from build123d import *

# Parameters (mm, degrees)
SKETCH1_W                        = 132.5
SKETCH1_H                        = 117
BOSS_EXTRUDE1_DEPTH              = 55.25
CUT_EXTRUDE1_REACH               = 147.364
SKETCH3_W                        = 39
SKETCH3_H                        = 37.83
CUT_EXTRUDE2_DEPTH               = 85
SKETCH4_W                        = 20.6
SKETCH4_H                        = 13
BOSS_EXTRUDE2_DEPTH              = 32
SKETCH5_W                        = 27.5
SKETCH5_H                        = 68.25
CUT_EXTRUDE3_DEPTH               = 3
SKETCH6_W                        = 46.9
SKETCH6_H                        = 3.4
CUT_EXTRUDE4_DEPTH               = 46.9
SKETCH8_R                        = 4.2
SKETCH8_R_2                      = 4.5
CUT_EXTRUDE5_DEPTH               = 14
SKETCH9_R                        = 14.58
CUT_EXTRUDE6_DEPTH               = 15.3
SKETCH10_R                       = 11.2
CUT_EXTRUDE7_DEPTH               = 7.22
BOSS_EXTRUDE3_DEPTH              = 4.25
CUT_EXTRUDE8_REACH               = 116.313
CUT_EXTRUDE8_END_RADIUS          = 4.2
SKETCH15_R                       = 2
F_4_0_MM_DOWEL_HOLES1_D          = 4
F_4_0_MM_DOWEL_HOLES2_AT_2_COUNT = 2
F_4_0_MM_DOWEL_HOLES2_AT_2_PITCH = 30
F_4_0_MM_DOWEL_HOLES3_D          = 4
F_4_0_MM_DOWEL_HOLES3_DEPTH      = 10
F_4_0_MM_DOWEL_HOLES3_TIP        = 1.201721238


with BuildPart() as part:
    # Sketch1 → Boss-Extrude1 (new body)
    with BuildSketch(Plane.XY):
        Rectangle(SKETCH1_W, SKETCH1_H)
    extrude(amount=BOSS_EXTRUDE1_DEPTH)

    # Sketch2 → Cut-Extrude1 (cut, up to next)
    with BuildSketch(Plane(origin=(0, 58.5, 0), x_dir=(1, 0, 0), z_dir=(0, 1, 0)), mode=Mode.PRIVATE) as cut_extrude1_sk1:
        with BuildLine():
            Line((-57.7, -32), (-57.7, -55.25))
            Line((-57.7, -55.25), (-22.3, -55.25))
            Line((-22.3, -55.25), (-22.3, -32))
            ThreePointArc((-22.3, -32), (-40, -14.3), (-57.7, -32))
        make_face()
    cut_extrude1_tool1 = extrude(cut_extrude1_sk1.sketch, amount=-CUT_EXTRUDE1_REACH, mode=Mode.PRIVATE) & part.part
    # Sketch2 → Cut-Extrude1 (cut, up to next)
    with BuildSketch(Plane(origin=(0, 58.5, 0), x_dir=(1, 0, 0), z_dir=(0, 1, 0)), mode=Mode.PRIVATE) as cut_extrude1_sk2:
        with BuildLine():
            Line((57.7, -32), (57.7, -55.25))
            Line((57.7, -55.25), (22.3, -55.25))
            Line((22.3, -55.25), (22.3, -32))
            ThreePointArc((22.3, -32), (40, -14.3), (57.7, -32))
        make_face()
    cut_extrude1_tool2 = extrude(cut_extrude1_sk2.sketch, amount=-CUT_EXTRUDE1_REACH, mode=Mode.PRIVATE) & part.part
    add(cut_extrude1_tool1.solids().sort_by_distance((-40, 58.5, 36.464181))[0], mode=Mode.SUBTRACT)
    add(cut_extrude1_tool2.solids().sort_by_distance((40, 58.5, 36.464181))[0], mode=Mode.SUBTRACT)

    # Sketch3 → Cut-Extrude2 (cut)
    with BuildSketch(Plane(origin=(0, 58.5, 0), x_dir=(1, 0, 0), z_dir=(0, 1, 0))):
        with Locations((0, -36.335)):
            Rectangle(SKETCH3_W, SKETCH3_H)
    extrude(amount=-CUT_EXTRUDE2_DEPTH, mode=Mode.SUBTRACT)

    # Sketch4 → Boss-Extrude2 (add)
    with BuildSketch(Plane(origin=(0, -26.5, 0), x_dir=(1, 0, 0), z_dir=(0, 1, 0))):
        with Locations((0, -61.75)):
            Rectangle(SKETCH4_W, SKETCH4_H)
    extrude(amount=-BOSS_EXTRUDE2_DEPTH)

    # Sketch5 → Cut-Extrude3 (cut)
    with BuildSketch(Plane.XZ.offset(58.5)):
        with Locations((0, 34.125)):
            Rectangle(SKETCH5_W, SKETCH5_H)
    extrude(amount=-CUT_EXTRUDE3_DEPTH, mode=Mode.SUBTRACT)

    # Sketch6 → Cut-Extrude4 (cut)
    with BuildSketch(Plane.XY.offset(55.25)):
        with Locations((-40, -54)):
            Rectangle(SKETCH6_W, SKETCH6_H)
        with Locations((40, -54)):
            Rectangle(SKETCH6_W, SKETCH6_H)
    extrude(amount=-CUT_EXTRUDE4_DEPTH, mode=Mode.SUBTRACT)

    # Sketch8 → Cut-Extrude5 (cut)
    with BuildSketch(Plane.XZ.offset(55.5)):
        with Locations(Location((0, 7, 0), (0, 0, 270))):
            Circle(SKETCH8_R)
        with Locations(Location((0, 57, 0), (0, 0, 270))):
            Circle(SKETCH8_R)
        with Locations(Location((0, 32, 0), (0, 0, 270))):
            Circle(SKETCH8_R_2)
    extrude(amount=-CUT_EXTRUDE5_DEPTH, mode=Mode.SUBTRACT)

    # Sketch9 → Cut-Extrude6 (cut)
    with BuildSketch(Plane(origin=(0, -26.5, 0), x_dir=(1, 0, 0), z_dir=(0, 1, 0))):
        with Locations(Location((0, -32, 0), (0, 0, 270))):
            Circle(SKETCH9_R)
    extrude(amount=-CUT_EXTRUDE6_DEPTH, mode=Mode.SUBTRACT)

    # Sketch10 → Cut-Extrude7 (cut)
    with BuildSketch(Plane(origin=(0, -41.8, 0), x_dir=(1, 0, 0), z_dir=(0, 1, 0))):
        with Locations(Location((0, -32, 0), (0, 0, 270))):
            Circle(SKETCH10_R)
    extrude(amount=-CUT_EXTRUDE7_DEPTH, mode=Mode.SUBTRACT)

    # Sketch12 → Ø3.5 (3.5) Diameter Hole1 (revolve, cut)
    with BuildSketch(Plane(origin=(0, -49.5, 68.25), x_dir=(0, -1, 0), z_dir=(1, 0, 0))):
        Polygon((0, 0), (0, 21.051506083), (1.75, 20), (1.75, 0), align=None)
    f_3_5_3_5_diameter_hole1 = revolve(axis=Axis((0, -49.5, 74.6), (0, 0, -1)), mode=Mode.SUBTRACT)

    # Sketch14 → Boss-Extrude3 (add)
    with BuildSketch(Plane(origin=(0, 0, 0), x_dir=(-1, 0, 0), z_dir=(0, 0, -1))):
        Polygon((-66.25, -58.5), (-13.75, -58.5), (-13.75, -55.5), (13.75, -55.5), (13.75, -58.5), (66.25, -58.5), (66.25, 58.5), (-66.25, 58.5), align=None)
    extrude(amount=BOSS_EXTRUDE3_DEPTH)

    # Cut-Extrude8: up to this cylinder (the profile starts outside it)
    cut_extrude8_end = Plane(origin=(0, -49.5, 57), z_dir=(0, -1, 0)) * Cylinder(CUT_EXTRUDE8_END_RADIUS, 242.026, mode=Mode.PRIVATE)
    # Sketch15 → Cut-Extrude8 (cut, up to the surface)
    with BuildSketch(Plane.XY.offset(68.25), mode=Mode.PRIVATE) as cut_extrude8_sk1:
        with Locations((0, -49.5)):
            Circle(SKETCH15_R)
    cut_extrude8_tool1 = extrude(cut_extrude8_sk1.sketch, amount=-CUT_EXTRUDE8_REACH, mode=Mode.PRIVATE) - cut_extrude8_end
    cut_extrude8 = cut_extrude8_tool1.solids().sort_by_distance((0, -49.5, 68.25))[0]
    add(cut_extrude8, mode=Mode.SUBTRACT)

    # Mirror1: Ø3.5 (3.5) Diameter Hole1, Cut-Extrude8 across plane
    add(f_3_5_3_5_diameter_hole1.mirror(Plane.XY.offset(32)), mode=Mode.SUBTRACT)
    add(cut_extrude8.mirror(Plane.XY.offset(32)), mode=Mode.SUBTRACT)

    # Ø4.0 mm Dowel Holes1 (through all)
    with Locations(Plane.XY.offset(17.42)):
        with Locations((-12.5, 32.58), (12.5, 32.58), (12.5, 44.58), (-12.5, 44.58)):
            Hole(F_4_0_MM_DOWEL_HOLES1_D / 2)

    # Sketch19 → Ø4.0 mm Dowel Holes2 (revolve, cut)
    with BuildSketch(Plane(origin=(61.975, -47.3, 55.25), x_dir=(0, -1, 0), z_dir=(1, 0, 0))):
        Polygon((0, 0), (0, 11.201721238), (2, 10), (2, 0), align=None)
    f_4_0_mm_dowel_holes2 = revolve(axis=Axis((61.975, -47.3, 61.6), (0, 0, -1)), mode=Mode.SUBTRACT)

    # Ø4.0 mm Dowel Holes2 at 2: Ø4.0 mm Dowel Holes2 ×2
    with Locations(*[(0, i * F_4_0_MM_DOWEL_HOLES2_AT_2_PITCH, 0) for i in range(1, F_4_0_MM_DOWEL_HOLES2_AT_2_COUNT)]):
        add(f_4_0_mm_dowel_holes2, mode=Mode.SUBTRACT)

    # Mirror2: Ø4.0 mm Dowel Holes2 across plane
    add(f_4_0_mm_dowel_holes2.mirror(Plane(origin=(0, 0, 0), x_dir=(0, 0, 1), z_dir=(1, 0, 0))), mode=Mode.SUBTRACT)

    # Mirror2 copy 1 sketch → Mirror2 copy 1 (revolve, cut)
    with BuildSketch(Plane(origin=(-61.975, -17.3, 55.25), x_dir=(0, -1, 0), z_dir=(-1, 0, 0))):
        Polygon((0, 0), (0, -11.201721238), (2, -10), (2, 0), align=None)
    revolve(axis=Axis((-61.975, -17.3, 61.6), (0, 0, 1)), mode=Mode.SUBTRACT)

    # Ø4.0 mm Dowel Holes3
    with Locations(Plane.XY.offset(68.25)):
        with Locations((0.2, -32.3)):
            Hole(F_4_0_MM_DOWEL_HOLES3_D / 2, depth=F_4_0_MM_DOWEL_HOLES3_DEPTH)
            with Locations((0, 0, -(F_4_0_MM_DOWEL_HOLES3_DEPTH + F_4_0_MM_DOWEL_HOLES3_TIP / 2))):  # 118° drill point
                Cone(0, F_4_0_MM_DOWEL_HOLES3_D / 2, F_4_0_MM_DOWEL_HOLES3_TIP, mode=Mode.SUBTRACT)


solid = part.part
Here's how the part is built. I have some questions about the finished solid (model axes, mm). A direction names the side the tool comes from. Coordinates: 2 decimals unless noted, no trailing zeros. Order: outer loops, then holes, each group sorted by start corner. A loop starts at its lowest first (then second) coordinate and runs counter-clockwise, first axis right, second up. Notation, with made-up numbers: (-13.75, 28.5) - (31.25, 28.5) arc R11 ccw to (31.25, 41.5) - close; hole circle Ø4 at (22, 36.5). An arc over 180 degrees is marked (long way). Use CSV: the item, a comma, the result in double quotes. Start each with the question number.
1. I'm going to push flat-ended pins straight in: pin 1 (5 mm diameter, centred on x = 12.5, y = 32.58, fed in from +Z); pin 2 (23.5 mm diameter, centred on x = 30, z = 36.5, fed in from +Y); pin 3 (6.5 mm diameter, centred on x = -1.5, z = 8.5, fed in from -Y); pin 4 (2.5 mm diameter, centred on x = 63, y = -15.5, fed in from +Z). Where does each tip first touch, or does it pass through?
2. Suppose I cut it at D-D on x = 24.5. List the corners of the cut face in (y, z) for me.
3. For faces 1 (the face through (-22.3, 4, 44)), 2 (the face through (-16.55, -54, 32)), 3 (the face through (19.5, 17, 37)), which set-ups out of +Z, -Z, +X, -X, +Y, -Y let a thin tool reach every point of the face, with its end or its side?
4. Suppose I cut it at B-B on x = -40. List the corners of the cut face in (y, z) for me.
5. Suppose I cut it at C-C on y = 7.5. List the corners of the cut face in (x, z) for me, then the cut area to 3 significant figures.
6. Suppose I cut it at A-A on y = 44.58. List the corners of the cut face in (x, z) for me.
7. Please list where these lines run through material, in increasing order: line 1 (X direction, y = 45.5, z = 34.5); line 2 (X direction, y = -17, z = 49); line 3 (Y direction, x = 12.5, z = 4). Write a range as from..to.
8. If we mould it in two halves opening along Y, with no side actions, what happens to faces 4 (the face through (-1.735, -49.272, 13.25)), 5 (the face through (57.7, 4, 43)), 6 (the face through (-63.19, -15.71, 50.32)), 7 (the face through (0, -26.5, 48))? For each: +Y half, -Y half, draft (parallel to the pull), parting line (faces both ways), or undercut.
Output:
1,pin 1,"stops at z = 17.42"
1,pin 2,"stops at y = 58.5"
1,pin 3,"stops at y = -55.5"
1,pin 4,"stops at z = 55.25"
2,outline,"(-58.5, -4.25) - (58.5, -4.25) - (58.5, 23.45) - (-52.3, 23.45) - (-52.3, 8.35) - (-55.7, 8.35) - (-55.7, 23.45) - (-58.5, 23.45) - close"
3,face 1,"+Z, +Y, -Y"
3,face 2,"+Z"
3,face 3,"+Z, +Y"
4,outline,"(-58.5, -4.25) - (58.5, -4.25) - (58.5, 14.3) - (-52.3, 14.3) - (-52.3, 8.35) - (-55.7, 8.35) - (-55.7, 14.3) - (-58.5, 14.3) - close"
5,outline,"(-66.25, -4.25) - (66.25, -4.25) - (66.25, 55.25) - (57.7, 55.25) - (57.7, 32) arc R17.7 cw to (22.3, 32) - (22.3, 55.25) - (19.5, 55.25) - (19.5, 17.42) - (-19.5, 17.42) - (-19.5, 55.25) - (-22.3, 55.25) - (-22.3, 32) arc R17.7 cw to (-57.7, 32) - (-57.7, 55.25) - (-66.25, 55.25) - close"
5,area,"3,780 mm2"
6,outline,"(-66.25, -4.25) - (-14.5, -4.25) - (-14.5, 17.42) - (-19.5, 17.42) - (-19.5, 55.25) - (-22.3, 55.25) - (-22.3, 32) arc R17.7 cw to (-57.7, 32) - (-57.7, 55.25) - (-66.25, 55.25) - close; (-10.5, -4.25) - (10.5, -4.25) - (10.5, 17.42) - (-10.5, 17.42) - close; (14.5, -4.25) - (66.25, -4.25) - (66.25, 55.25) - (57.7, 55.25) - (57.7, 32) arc R17.7 cw to (22.3, 32) - (22.3, 55.25) - (19.5, 55.25) - (19.5, 17.42) - (14.5, 17.42) - close"
7,line 1,"x = -66.25..-57.7, -22.3..-19.5, 19.5..22.3, 57.7..66.25"
7,line 2,"x = -66.25..-63.95, -60..-57.7, -22.3..-19.5, 19.5..22.3, 57.7..60, 63.95..66.25"
7,line 3,"y = -55.5..30.58, 34.58..42.58, 46.58..58.5"
8,face 4,"undercut"
8,face 5,"draft"
8,face 6,"undercut"
8,face 7,"+Y half"
